Geometry: final body of the model. Coordinates: model frame, mm. A direction names the side the tool comes from. Round coordinates to 2 decimals unless told otherwise and drop trailing zeros. Order: outer loops, then holes, each group sorted by start corner. A loop starts at its lowest first (then second) coordinate and runs counter-clockwise, first axis right, second up. Notation, with made-up numbers: M 42.25,-0.5 L 71.25,-0.5 A23 cw 71.25,27.5 Z; hole C 26,12.5 d2. An arc over 180 degrees is marked long. Put each result on its own line as item: value. Start each with the question number.
1) Section B-B, the plane y = 5.5. Return loops of the section in (x, z).
2) Section C-C, the plane z = -2.5. Return loops of the section in (x, y), then the cut area to 3 significant figures.
3) Access query for faces 4 (the flat face through (13, 7, 1)), 5 (the cylindrical face through (23.4, 6.85, -0.57)), 6 (the flat face through (13, 5, 2)). Directions: +Z, -Z, +X, -X, +Y, -Y. A direction counts if a zero-diameter tool reaches every point of the face in a straight line with its end or side. Return the directions, or none.
4) Draft query along X for faces 1 (the cylindrical face through (1.203, 5.121, 0.859)), 2 (the flat face through (24.4, 10.1, -28.7)), 3 (the flat face through (3, 7, -21)). Return one class per face: pulls with the +X half, pulls with the -X half, needs draft (parallel to the pull), parting line crosses it, or undercut.
5) Material intervals for probe 1 along X at (y, z) = (5, -45.3); probe 2 along Z at (x, y) = (15, 6.5); probe 3 along Y at (x, z) = (7.25, -11.5), sorted ascending. Write a range as [from, to].
6) Section D-D, the plane x = 13.5. Return loops of the section in (y, z), then the cut area to 3 significant figures.
7) Section A-A, the plane x = 18. Return loops of the section in (y, z), then the cut area to 3 significant figures.
8) First-contact query: P1, Ø1.6, axis at y = 8.5, z = 1.5, coming from the +X side; P2, Ø10, axis at x = 7.5, y = -2, coming from the -Z side; P3, Ø10.5, axis at x = 16, z = -19, coming from the +Y side; P4, Ø6, axis at x = 8.5, z = -24, coming from the -Y side. Flat tips, straight axial feed; report the tip coordinate or a pass-through.
from build123d import *

# Parameters (mm, degrees)
SKETCH1_W           = 27
SKETCH1_H           = 41
BOSS_EXTRUDE1_DEPTH = 3.5
SKETCH2_W           = 3
SKETCH2_H           = 41
BOSS_EXTRUDE2_DEPTH = 7.5
SKETCH3_R           = 4
BOSS_EXTRUDE3_DEPTH = 10
SKETCH4_W           = 27
SKETCH4_H           = 11
BOSS_EXTRUDE4_DEPTH = 2
SKETCH5_W           = 27
SKETCH5_H           = 11
BOSS_EXTRUDE5_DEPTH = 2
CUT_EXTRUDE1_REACH  = 55.619
SKETCH6_W           = 7
SKETCH6_H           = 4
SKETCH7_W           = 27
SKETCH7_H           = 11
BOSS_EXTRUDE6_DEPTH = 5
SKETCH8_R           = 1.75
CUT_EXTRUDE2_DEPTH  = 59.940648113
SKETCH9_W           = 27
SKETCH9_H           = 50
CUT_EXTRUDE3_DEPTH  = 0.9
FILLET1_R           = 4
FILLET2_R           = 2


with BuildPart() as part:
    # Sketch1 → Boss-Extrude1 (new body)
    with BuildSketch(Plane(origin=(0, 0, 0), x_dir=(1, 0, 0), z_dir=(0, 1, 0))):
        with Locations((13.5, 20.5)):
            Rectangle(SKETCH1_W, SKETCH1_H)
    extrude(amount=BOSS_EXTRUDE1_DEPTH)

    # Sketch2 → Boss-Extrude2 (add)
    with BuildSketch(Plane(origin=(0, 3.5, 0), x_dir=(1, 0, 0), z_dir=(0, 1, 0))):
        with Locations((1.5, 20.5)):
            Rectangle(SKETCH2_W, SKETCH2_H)
        with Locations((25.5, 20.5)):
            Rectangle(SKETCH2_W, SKETCH2_H)
    extrude(amount=BOSS_EXTRUDE2_DEPTH)

    # Sketch3 → Boss-Extrude3 (add)
    with BuildSketch(Plane(origin=(0, 0, 0), x_dir=(-1, 0, 0), z_dir=(0, -1, 0))):
        with Locations(Location((-13.5, 10, 0), (0, 0, 270))):
            Circle(SKETCH3_R)
    extrude(amount=BOSS_EXTRUDE3_DEPTH)

    # Sketch4 → Boss-Extrude4 (add)
    with BuildSketch(Plane(origin=(0, 0, -41), x_dir=(-1, 0, 0), z_dir=(0, 0, -1))):
        with Locations((-13.5, 5.5)):
            Rectangle(SKETCH4_W, SKETCH4_H)
    extrude(amount=BOSS_EXTRUDE4_DEPTH)

    # Sketch5 → Boss-Extrude5 (add)
    with BuildSketch(Plane.XY):
        with Locations((13.5, 5.5)):
            Rectangle(SKETCH5_W, SKETCH5_H)
    extrude(amount=BOSS_EXTRUDE5_DEPTH)

    # Sketch6 → Cut-Extrude1 (cut, up to next)
    with BuildSketch(Plane.XY.offset(2), mode=Mode.PRIVATE) as cut_extrude1_sk1:
        with Locations((13.5, 9)):
            Rectangle(SKETCH6_W, SKETCH6_H)
    cut_extrude1_tool1 = extrude(cut_extrude1_sk1.sketch, amount=-CUT_EXTRUDE1_REACH, mode=Mode.PRIVATE) & part.part
    add(cut_extrude1_tool1.solids().sort_by_distance((13.5, 9, 2))[0], mode=Mode.SUBTRACT)

    # Sketch7 → Boss-Extrude6 (add)
    with BuildSketch(Plane(origin=(0, 0, -43), x_dir=(-1, 0, 0), z_dir=(0, 0, -1))):
        with Locations((-13.5, 5.5)):
            Rectangle(SKETCH7_W, SKETCH7_H)
    extrude(amount=BOSS_EXTRUDE6_DEPTH)

    # Sketch8 → Cut-Extrude2 (cut, through all)
    with BuildSketch(Plane(origin=(0, 11, 0), x_dir=(1, 0, 0), z_dir=(0, 1, 0))):
        with Locations(Location((18, 45.3, 0), (0, 0, 270))):
            Circle(SKETCH8_R)
        with Locations(Location((9, 45.3, 0), (0, 0, 270))):
            Circle(SKETCH8_R)
    extrude(amount=-CUT_EXTRUDE2_DEPTH, mode=Mode.SUBTRACT)

    # Sketch9 → Cut-Extrude3 (cut)
    with BuildSketch(Plane(origin=(0, 11, 0), x_dir=(1, 0, 0), z_dir=(0, 1, 0))):
        with Locations((13.5, 23)):
            Rectangle(SKETCH9_W, SKETCH9_H)
    extrude(amount=-CUT_EXTRUDE3_DEPTH, mode=Mode.SUBTRACT)

    # Fillet1
    fillet1_edges = [part.edges().sort_by_distance(p)[0] for p in [
        (27, 5.05, -48),
        (0, 5.05, 2),
        (27, 5.05, 2),
        (0, 5.05, -48),
    ]]
    fillet(fillet1_edges, radius=FILLET1_R)

    # Fillet2
    fillet2_edges = [part.edges().sort_by_distance(p)[0] for p in [
        (24, 6.8, 0),
        (3, 6.8, 0),
    ]]
    fillet(fillet2_edges, radius=FILLET2_R)


solid = part.part
Result sheet:
1. outline: M 0,-44 A4 ccw 4,-48 L 23,-48 A4 ccw 27,-44 L 27,-2 A4 ccw 23,2 L 4,2 A4 ccw 0,-2 Z; hole M 3,-41 L 24,-41 L 24,-2 A2 ccw 22,0 L 5,0 A2 ccw 3,-2 Z; hole C 9,-45.3 d3.5; hole C 18,-45.3 d3.5
2. outline: M 0,0 L 27,0 L 27,10.1 L 24,10.1 L 24,3.5 L 3,3.5 L 3,10.1 L 0,10.1 Z
2. area: 134 mm2
3. face 4: +Z, +Y
3. face 5: +Y
3. face 6: +Z, +X, -X, +Y, -Y
4. face 1: pulls with the -X half
4. face 2: needs draft
4. face 3: undercut
5. probe 1: x = [0.22, 7.25], [10.75, 16.25], [19.75, 26.78]
5. probe 2: z = [-48, -41], [0, 2]
5. probe 3: y = [0, 3.5]
6. outline: M -10,-14 L 0,-14 L 0,-48 L 10.1,-48 L 10.1,-41 L 3.5,-41 L 3.5,0 L 7,0 L 7,2 L 0,2 L 0,-6 L -10,-6 Z
6. area: 308 mm2
7. outline: M 0,-48 L 10.1,-48 L 10.1,-47.05 L 0,-47.05 Z; M 0,-43.55 L 10.1,-43.55 L 10.1,-41 L 3.5,-41 L 3.5,0 L 10.1,0 L 10.1,2 L 0,2 Z
7. area: 199 mm2
8. P1: stops at x = 25.95
8. P2: stops at z = -48
8. P3: stops at y = 3.5
8. P4: stops at y = 0
